The listing builds one solid part. Answer for the finished solid, in the listing's coordinates (mm). Face numbers are marked on the shaded views. Coordinates: 2 decimals unless noted, no trailing zeros. Write each loop counter-clockwise with the first axis right and the second up, starting at its lowest first coordinate (ties: lowest second). Pieces come first, ordered by that corner, then holes.
```python
from build123d import *

# Parameters (mm, degrees)
CROQUIS2_R            = 2.5
CORTAR_EXTRUIR1_DEPTH = 15
MATRIZC1_COUNT        = 3


with BuildPart() as part:
    # Croquis1 → Revolución1 (revolve)
    with BuildSketch(Plane(origin=(0, 0, 0), x_dir=(0, 0, -1), z_dir=(1, 0, 0))):
        Polygon((-95, 14), (-95, 12), (-40, 12), (-40, 0), (65, 0), (65, 10), (-15, 10), (-15, 14), align=None)
    revolve(axis=Axis((0, 0, 144.04817275), (0, 0, -1)))

    # Croquis2 → Cortar-Extruir1 (cut)
    with BuildSketch(Plane(origin=(0, 0, 0), x_dir=(1, 0, 0), z_dir=(0, 1, 0))):
        with Locations((0, -83)):
            Circle(CROQUIS2_R)
        with Locations((0, -57)):
            Circle(CROQUIS2_R)
    cortar_extruir1 = extrude(amount=-CORTAR_EXTRUIR1_DEPTH, mode=Mode.SUBTRACT)

    # MatrizC1: Cortar-Extruir1 ×3 about axis
    matrizc1_axis = Axis((0, 0, 103), (0, 0, -1))
    for i in range(1, MATRIZC1_COUNT):
        add(cortar_extruir1.rotate(matrizc1_axis, i * 360 / MATRIZC1_COUNT), mode=Mode.SUBTRACT)


solid = part.part
```
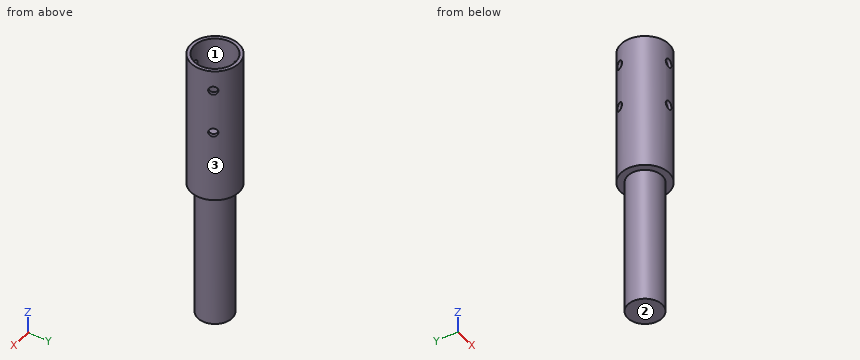
(1) Section B-B, the plane z = 83 is taken. Write down the section's boundary in (x, y), plus the area to 3 significant figures.
(2) Section C-C, the plane y = 0 is taken. Write down the section's boundary in (x, z).
(3) For a pull along X with two mould halves and no side action, classify the marked faces 1, 2 and 3 as pulls with the +X half, pulls with the -X half, needs draft (parallel to the pull), parting line crosses it, or undercut.
(4) Each of these flat-tipped pins is pushed along its axis until it touches: pin 1 (1.5 mm diameter, centred on y = 3, z = 12.5, fed in from +X); pin 2 (6 mm diameter, centred on y = 10, z = 52, fed in from -X); pin 3 (4 mm diameter, centred on x = 3.5, z = 38.5, fed in from +Y). Where does it stop, or does it pass through?
(5) Find the intervals of material crossed by probe 1 along X at (y, z) = (0, 54); probe 2 along Y at (x, z) = (-0.75, 60.5); probe 3 along Z at (x, y) = (10.75, -2.75), in increasing order.
(6) Section A-A, the plane x = 0 is taken. Write down the section's boundary in (y, z).
(7) Section D-D, the plane z = 52.5 is taken. Write down the section's boundary in (x, y), plus the area to 3 significant figures.
Solution:
1. outline: (-13.18, 4.72) arc R14 ccw to (-2.5, -13.77) - (-2.5, -11.74) arc R12 cw to (-11.41, 3.7) - close; (-10.68, 9.05) - (-8.91, 8.03) arc R12 cw to (8.91, 8.03) - (10.68, 9.05) arc R14 ccw to start; (2.5, -13.77) arc R14 ccw to (13.18, 4.72) - (11.41, 3.7) arc R12 cw to (2.5, -11.74) - close
1. area: 133 mm2
2. outline: (-14, 15) - (-10, 15) - (-10, -65) - (10, -65) - (10, 15) - (14, 15) - (14, 95) - (12, 95) - (12, 40) - (-12, 40) - (-12, 95) - (-14, 95) - close
3. face 1: undercut
3. face 2: needs draft
3. face 3: parting line crosses it
4. pin 1: stops at x = 9.74
4. pin 2: stops at x = -12.12
4. pin 3: stops at y = 13.92
5. probe 1: x = -14 to -12, 12 to 14
5. probe 2: y = -13.98 to -11.98, 11.98 to 13.98
5. probe 3: z = 15 to 40
6. outline: (-14, 15) - (-10, 15) - (-10, -65) - (10, -65) - (10, 15) - (14, 15) - (14, 95) - (12, 95) - (12, 40) - (-12, 40) - (-12, 54.5) - (-14, 54.5) - close; (-14, 59.5) - (-12, 59.5) - (-12, 80.5) - (-14, 80.5) - close; (-14, 85.5) - (-12, 85.5) - (-12, 95) - (-14, 95) - close
7. outline: circle Ø28 at (0, 0); hole circle Ø24 at (0, 0)
7. area: 163 mm2
